Here's how the part is built. I have some questions about the finished solid (model axes, mm). A direction names the side the tool comes from. Coordinates: 2 decimals unless noted, no trailing zeros. Loops run counter-clockwise (first coordinate to the right, second up) from the corner with the lowest first, then second, coordinate; pieces in that order, holes last.
```python
from build123d import *

# Parameters (mm, degrees)
SCHIZZO1_W                   = 35.931818182
SCHIZZO1_H                   = 10.2
SCHIZZO1_W_2                 = 33
SCHIZZO1_H_2                 = 7.2
ESTRUSIONE_ESTRUSIONE1_DEPTH = 330
SCHIZZO3_W                   = 2.7
SCHIZZO3_H                   = 3.2
TAGLIO_ESTRUSIONE1_DEPTH     = 34.465909091
TAGLIO_ESTRUSIONE2_DEPTH     = 1.5
SMUSSO2_SIZE                 = 0.6
SCHIZZO5_W                   = 49.931818182
SCHIZZO5_H                   = 24.2
SCHIZZO5_W_2                 = 35.931818182
SCHIZZO5_H_2                 = 10.2
ESTRUSIONE_ESTRUSIONE2_DEPTH = 2


with BuildPart() as part:
    # Schizzo1 → Estrusione-Estrusione1 (new body)
    with BuildSketch(Plane.XY):
        Rectangle(SCHIZZO1_W, SCHIZZO1_H)
        Rectangle(SCHIZZO1_W_2, SCHIZZO1_H_2, mode=Mode.SUBTRACT)
    extrude(amount=ESTRUSIONE_ESTRUSIONE1_DEPTH)

    # Schizzo3 → Taglio-Estrusione1 (cut)
    with BuildSketch(Plane.ZY.offset(17.965909091)):
        with Locations((4.35, 2)):
            Rectangle(SCHIZZO3_W, SCHIZZO3_H)
    extrude(amount=-TAGLIO_ESTRUSIONE1_DEPTH, mode=Mode.SUBTRACT)

    # Schizzo4 → Taglio-Estrusione2 (cut)
    with BuildSketch(Plane(origin=(0, 5.1, 0), x_dir=(1, 0, 0), z_dir=(0, 1, 0))):
        with BuildLine():
            Line((-16.5, -5.45), (15.4, -5.45))
            ThreePointArc((15.4, -5.45), (16.5, -4.35), (15.4, -3.25))
            Line((15.4, -3.25), (-16.5, -3.25))
            Line((-16.5, -3.25), (-16.5, -3))
            Line((-16.5, -3), (-17.965909091, -3))
            Line((-17.965909091, -3), (-17.965909091, -5.7))
            Line((-17.965909091, -5.7), (-16.5, -5.7))
            Line((-16.5, -5.7), (-16.5, -5.45))
        make_face()
    extrude(amount=-TAGLIO_ESTRUSIONE2_DEPTH, mode=Mode.SUBTRACT)

    # Smusso2
    smusso2_edges = [part.edges().sort_by_distance(p)[0] for p in [
        (-0.55, 5.1, 3.25),
        (16.5, 5.1, 4.35),
        (-0.55, 5.1, 5.45),
    ]]
    chamfer(smusso2_edges, length=SMUSSO2_SIZE)

    # Schizzo5 → Estrusione-Estrusione2 (add)
    with BuildSketch(Plane(origin=(0, 0, 0), x_dir=(-1, 0, 0), z_dir=(0, 0, -1))):
        Rectangle(SCHIZZO5_W, SCHIZZO5_H)
        Rectangle(SCHIZZO5_W_2, SCHIZZO5_H_2, mode=Mode.SUBTRACT)
    extrude(amount=-ESTRUSIONE_ESTRUSIONE2_DEPTH)


solid = part.part
```
1. I want a section at A-A (x = -6.5). Please give me the cut outline in (y, z).
2. On a 3-axis mill with a long thin cutter (end or side, diameter ignored), from which of +Z, -Z, +X, -X, +Y, -Y can I reach the whole of each face in a straight line? I mean faces 1 (the flat face through (0, -5.1, 164)), 2 (the flat face through (-17.966, 0, 164)), 3 (the flat face through (16.5, 0, 163)). Say none if no direction works.
3. I want a section at B-B (z = 118). Please give me the cut outline in (x, y).
4. For pin 1 (6 mm diameter, centred on y = 1, z = 224, fed in from +X); pin 2 (5 mm diameter, centred on y = 2, z = 125.5, fed in from -X); pin 3 (1 mm diameter, centred on x = 10.5, z = 135, fed in from +Y), each with a flat end and sliding along its axis, tell me the tip position at first contact or that it passes through.
5. I need wall thicknesses on line 1 along Y through (x, z) = (4.5, 150.5); line 2 along X through (y, z) = (2.5, 22); line 3 along Z through (x, y) = (16, -9). Which ranges of each line are inside material? Lowest first, please.
6. We'd pull the mould along X, two halves only. Please class faces 4 (the flat face through (0, -3.6, 163)), 5 (the flat face through (17.966, 0, 164)), 6 (the flat face through (0, 4, 330)): +X half, -X half, draft (parallel to the pull), parting line (faces both ways), or undercut.
Response values:
1. outline: (-12.1, 0) - (-3.6, 0) - (-3.6, 330) - (-5.1, 330) - (-5.1, 2) - (-12.1, 2) - close; (3.6, 0) - (12.1, 0) - (12.1, 2) - (5.1, 2) - (5.1, 2.65) - (4.5, 3.25) - (3.6, 3.25) - close; (3.6, 5.45) - (4.5, 5.45) - (5.1, 6.05) - (5.1, 330) - (3.6, 330) - close
2. face 1: +Z, +X, -X, -Y
2. face 2: +Z, -X, +Y, -Y
2. face 3: +Z, -Z
3. outline: (-17.97, -5.1) - (17.97, -5.1) - (17.97, 5.1) - (-17.97, 5.1) - close; hole (-16.5, -3.6) - (16.5, -3.6) - (16.5, 3.6) - (-16.5, 3.6) - close
4. pin 1: stops at x = 17.97
4. pin 2: stops at x = -17.97
4. pin 3: stops at y = 5.1
5. line 1: y = -5.1 to -3.6, 3.6 to 5.1
5. line 2: x = -17.97 to -16.5, 16.5 to 17.97
5. line 3: z = 0 to 2
6. face 4: undercut
6. face 5: +X half
6. face 6: draft
